For this review, take the finished solid that the model builds, in its own axes (mm). Face numbers are marked on the shaded views. A direction names the side the tool comes from. Give positions to 0.01 mm unless a question says otherwise; leave off trailing zeros. Write each loop counter-clockwise with the first axis right and the second up, starting at its lowest first coordinate (ties: lowest second). Pieces come first, ordered by that corner, then holes.
1) Machinability: for the marked faces 4 and 5, which of the approach directions +Z, -Z, +X, -X, +Y, -Y give a long, thin tool a straight path to every point of the face, cutting with its end or side? Answer none if there is none.
2) For P1, Ø5, axis at y = 102.5, z = 16.5, coming from the -X side; P2, Ø5.5, axis at x = 222, y = 101.5, coming from the +Z side; P3, Ø1.5, axis at y = 101, z = 9.5, coming from the +X side, all flat-tipped, find the tip position at first contact; note any pin that passes through.
3) We need section C-C on z = 22. Give the boundary of the cut face in (x, y).
4) We need section A-A on x = 235. Give the boundary of the cut face in (y, z), and give its area (3 significant figures).
5) Wall thickness on line 1 along Y through (x, z) = (233.5, 13.5); line 2 along Z through (x, y) = (242.5, 108); line 3 along Y through (x, z) = (196, 14): over which ranges is each line inside the solid? List them lowest first.
6) We need section B-B on y = 105.25. Give the boundary of the cut face in (x, z).
7) We need section D-D on x = 196.5. Give the boundary of the cut face in (y, z).
8) Draft analysis for pull direction Y (two halves, no side actions). For the marked faces 1, 2 and 3, state which applies: pulls with the +Y half, pulls with the -Y half, needs draft (parallel to the pull), parting line crosses it, or undercut.
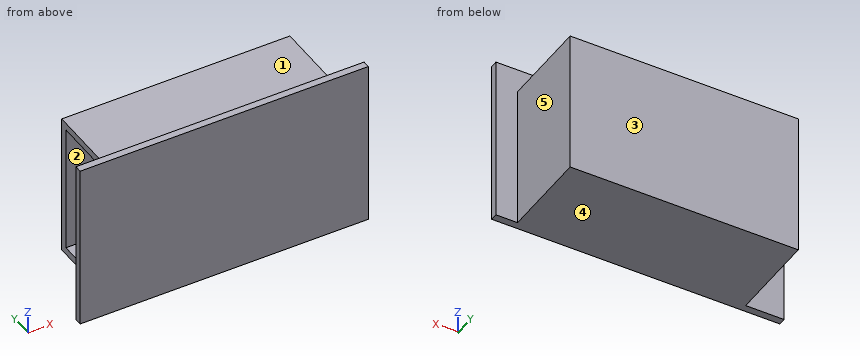
from build123d import *

# Parameters (mm, degrees)
BOX038_W     = 60
BOX038_H     = 1.5
BOX038_DEPTH = 35
BOX037_W     = 47.5
BOX037_H     = 17.2
BOX037_DEPTH = 27
BOX036_W     = 47.5
BOX036_H     = 18.7
BOX036_DEPTH = 30


with BuildPart() as cube038:
    # Box038 → Box038 (new body)
    with BuildSketch(Plane(origin=(192, 89.5, 0), x_dir=(1, 0, 0), z_dir=(0, 0, 1))):
        with Locations((30, 0.75)):
            Rectangle(BOX038_W, BOX038_H)
    extrude(amount=BOX038_DEPTH)


with BuildPart() as cube037:
    # Box037 → Box037 (new body)
    with BuildSketch(Plane(origin=(-1.5, 0, 60), x_dir=(1, 0, 0), z_dir=(0, 0, 1))):
        with Locations((23.75, 8.6)):
            Rectangle(BOX037_W, BOX037_H)
    extrude(amount=BOX037_DEPTH)


with BuildPart() as batteryholdertest:
    # Box036 → Box036 (new body)
    with BuildSketch(Plane.XY.offset(58.5)):
        with Locations((23.75, 9.35)):
            Rectangle(BOX036_W, BOX036_H)
    extrude(amount=BOX036_DEPTH)

    # Cut045: cut Cube037
    add(cube037.part, mode=Mode.SUBTRACT)


with BuildPart() as batteryholdertest_1:
    # Cut045 placement: moved
    add(batteryholdertest.part.moved(Location((200, 91, -58.5))))

    # Connect004: union Cube038
    add(cube038.part)


solid = batteryholdertest_1.part
Results list:
1. face 4: -Z, +X, -X, +Y, -Y
1. face 5: +Z, -Z, +X, +Y
2. P1: stops at x = 246
2. P2: stops at z = 30
2. P3: stops at x = 247.5
3. outline: (192, 89.5) - (252, 89.5) - (252, 91) - (247.5, 91) - (247.5, 109.7) - (200, 109.7) - (200, 108.2) - (246, 108.2) - (246, 91) - (192, 91) - close
4. outline: (89.5, 0) - (109.7, 0) - (109.7, 30) - (91, 30) - (91, 35) - (89.5, 35) - close; hole (91, 1.5) - (108.2, 1.5) - (108.2, 28.5) - (91, 28.5) - close
4. area: 149 mm2
5. line 1: y = 89.5 to 91, 108.2 to 109.7
5. line 2: z = 0 to 1.5, 28.5 to 30
5. line 3: y = 89.5 to 91
6. outline: (200, 0) - (247.5, 0) - (247.5, 30) - (200, 30) - (200, 28.5) - (246, 28.5) - (246, 1.5) - (200, 1.5) - close
7. outline: (89.5, 0) - (91, 0) - (91, 35) - (89.5, 35) - close
8. face 1: needs draft
8. face 2: undercut
8. face 3: pulls with the +Y half
